from build123d import *

# Parameters (mm, degrees)
F0_R     = 4.65
F1_DEPTH = 14.5
F2_R     = 4
F3_DEPTH = 10
F4_R     = 2
F5_DEPTH = 17
F6_R     = 3.5
F7_DEPTH = 2
F8_R     = 2.45
F9_DEPTH = 6.2


with BuildPart() as f1:
    # F0 (on Top) → F1 (new body)
    with BuildSketch(Plane.XY):
        Circle(F0_R)
    extrude(amount=F1_DEPTH)

    # F2 (on face) → F3 (join)
    with BuildSketch(Plane.XY.offset(14.5)):
        Circle(F2_R)
    extrude(amount=F3_DEPTH)

    # F4 (on face) → F5 (cut)
    with BuildSketch(Plane.XY.offset(24.5)):
        Circle(F4_R)
    extrude(amount=-F5_DEPTH, mode=Mode.SUBTRACT)

    # F6 (on face) → F7 (join)
    with BuildSketch(Plane(origin=(0, 0, 0), x_dir=(1, 0, 0), z_dir=(0, 0, -1))):
        Circle(F6_R)
    extrude(amount=F7_DEPTH)

    # F8 (on face) → F9 (join)
    with BuildSketch(Plane(origin=(0, 0, -2), x_dir=(1, 0, 0), z_dir=(0, 0, -1))):
        Circle(F8_R)
    extrude(amount=F9_DEPTH)


solid = f1.part
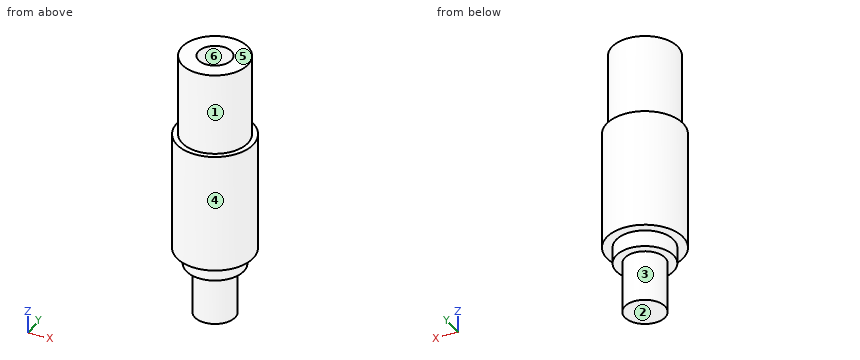
Work out the finished part from the listing and answer in its coordinate system (mm). Face numbers are marked on the shaded views. A direction names the side the tool comes from. Coordinates: 2 decimals unless noted, no trailing zeros. Write each loop counter-clockwise with the first axis right and the second up, starting at its lowest first coordinate (ties: lowest second). Pieces come first, ordered by that corner, then holes.
1. The part is cut by section C-C, the plane z = 21. Write down the section's boundary in (x, y).
Results list:
outline: circle Ø8 at (0, 0); hole circle Ø4 at (0, 0)
2. The part is cut by section A-A, the plane y = 0. Write down the section's boundary in (x, z), and give its area (3 significant figures).
Results list:
outline: (-4.65, 0) - (-3.5, 0) - (-3.5, -2) - (-2.45, -2) - (-2.45, -8.2) - (2.45, -8.2) - (2.45, -2) - (3.5, -2) - (3.5, 0) - (4.65, 0) - (4.65, 14.5) - (4, 14.5) - (4, 24.5) - (2, 24.5) - (2, 7.5) - (-2, 7.5) - (-2, 24.5) - (-4, 24.5) - (-4, 14.5) - (-4.65, 14.5) - close
area: 191 mm2
3. Consider line 1 along Y through (x, z) = (0, 12.5); line 2 along Y through (x, z) = (0, 19.25); line 3 along X through (y, z) = (0, -4). Determine where each line is inside the solid, lowest interval first.
Results list:
line 1: y = -4.65 to -2, 2 to 4.65
line 2: y = -4 to -2, 2 to 4
line 3: x = -2.45 to 2.45
4. For a pull along X with two mould halves and no side action, classify the marked faces 4, 5 and 6 as +X half, -X half, draft (parallel to the pull), parting line (faces both ways), or undercut.
Results list:
face 4: parting line
face 5: draft
face 6: undercut
5. The part is cut by section D-D, the plane z = 14. Write down the section's boundary in (x, y), and give its area (3 significant figures).
Results list:
outline: circle Ø9.3 at (0, 0); hole circle Ø4 at (0, 0)
area: 55.4 mm2
6. Flat-ended cylindrical pins translate along their axes: pin 1 (1.5 mm diameter, centred on y = 3.5, z = -2.5, fed in from -X); pin 2 (1 mm diameter, centred on x = -3.5, z = -3.5, fed in from -Y). Find the tip coordinate at first contact, or state that the pin passes through.
Results list:
pin 1: stops at x = -1.9
pin 2: passes through
7. For the marked faces 1, 2 and 3, determine the directions among +Z, -Z, +X, -X, +Y, -Y from which every point of the face is accessible in a straight line to the end or side of a thin tool.
Results list:
face 1: +Z
face 2: -Z, +X, -X, +Y, -Y
face 3: -Z
